Build history of the part. All positions in model axes, mm. A direction names the side the tool comes from. Give positions to 0.01 mm unless a question says otherwise; leave off trailing zeros. Order: outer loops, then holes, each group sorted by start corner. A loop starts at its lowest first (then second) coordinate and runs counter-clockwise, first axis right, second up. Notation, with made-up numbers: (61.5, 5.25) -> (79.5, 5.25) arc R11 ccw to (79.5, 25.25) -> close; hole circle Ø6 at (33, 40). An arc over 180 degrees is marked (long way). One line per question, with ' | ' between items. Start each with the question number.
(1) Which spindle directions (+Z, -Z, +X, -X, +Y, -Y) get a long thin tool onto all of the face, cutting with end or side? Do faces 4 (the face through (-378.557, 220, -53)), 5 (the face through (-403.957, 307, -329)), 6 (the face through (262, 68.014, -329)), 7 (the face through (201, -474.911, -329)), 8 (the face through (-365.857, 299, -543)). Say none if no direction does.
(2) Cut at A-A (z = -505). Give the cut face in (x, y).
(3) Cut at D-D (y = -302). Give the cut face in (x, z) (3 decimals).
(4) Cut at B-B (y = 164). Give the cut face in (x, z) (3 decimals), then the cut area to 3 significant figures.
(5) Cut at C-C (x = 76.5). Give the cut face in (y, z) (3 decimals).
(6) Drill centre lines: L1, parallel to Z at x = -89, y = 190 (3 decimals); L2, parallel to X at y = 117.5, z = -301; L3, parallel to Y at x = -385, z = -270.5. Where is each one in solid material? Low to high. Write a range as from..to.
(7) Pull direction Y, two halves, no side cores. Call faces 1 (the face through (291, -465.386, -53)), 2 (the face through (181.619, -366, -409)), 3 (the face through (-394.432, 218, -53)): +Y half, -Y half, draft (parallel to the pull), parting line (faces both ways), or undercut.
(8) Pin check, flat tips, straight feed: pin 1 Ø8 at (x, z) = (53, -203.5) entering from -Y; pin 2 Ø11.5 at (x, z) = (208, -504) entering from +Y; pin 3 Ø6 at (y, z) = (-282, -225) entering from -X. Stop position of each tip, or through.
from build123d import *

# Parameters (mm, degrees)
F1_DEPTH  = 15.875
F3_DEPTH  = 666.75
F4_W      = 139.7
F4_H      = 266.7
F4_H_2    = 244.475
F5_DEPTH  = 25.4
F6_W      = 139.7
F6_H      = 47.625
F7_DEPTH  = 12.7
F8_W      = 139.7
F8_H      = 47.625
F9_DEPTH  = 12.7
F10_W     = 139.7
F10_H     = 266.7
F10_H_2   = 244.475
F11_DEPTH = 25.4
F12_W     = 139.7
F12_H     = 47.625
F13_DEPTH = 12.7
F14_W     = 139.7
F14_H     = 47.625
F15_DEPTH = 12.7
F17_DEPTH = 504.825
F19_DEPTH = 504.825
F21_DEPTH = 3.175


with BuildPart() as f1:
    # F0 (on Top) → F1 (new body)
    with BuildSketch(Plane.XY):
        Polygon((177.06789, 329.740763), (-419.83211, 329.740763), (-419.83211, 88.440763), (159.394409, -490.785757), (400.694409, -490.785757), (400.694409, 106.114243), align=None)
    extrude(amount=F1_DEPTH)

    # F2 (on face) → F3 (join)
    with BuildSketch(Plane(origin=(0, 0, 0), x_dir=(1, 0, 0), z_dir=(0, 0, -1))):
        Polygon((397.519409, 436.810757), (397.519409, 474.910757), (359.419409, 474.910757), (359.419409, 465.385757), (219.719409, 465.385757), (219.719409, 474.910757), (181.619409, 474.910757), (181.619409, 436.810757), (219.719409, 436.810757), (219.719409, 449.510757), (359.419409, 449.510757), (359.419409, 436.810757), (381.644409, 436.810757), align=None)
        Polygon((397.519409, -83.889243), (397.519409, 436.810757), (381.644409, 436.810757), (381.644409, -68.014243), (138.96789, -68.014243), (138.96789, -310.690763), (-365.85711, -310.690763), (-365.85711, -326.565763), (154.84289, -326.565763), (154.84289, -310.690763), (154.84289, -83.889243), (381.644409, -83.889243), align=None)
        Polygon((-365.85711, -326.565763), (-365.85711, -310.690763), (-365.85711, -288.465763), (-378.55711, -288.465763), (-378.55711, -148.765763), (-365.85711, -148.765763), (-365.85711, -110.665763), (-403.95711, -110.665763), (-403.95711, -148.765763), (-394.43211, -148.765763), (-394.43211, -288.465763), (-403.95711, -288.465763), (-403.95711, -326.565763), align=None)
    extrude(amount=F3_DEPTH)

    # F4 (on face) → F5 (cut)
    with BuildSketch(Plane(origin=(-394.43211, 0, 0), x_dir=(0, -1, 0), z_dir=(-1, 0, 0))):
        with Locations((-218.615763, -241.3)):
            Rectangle(F4_W, F4_H)
        with Locations((-218.615763, -544.5125)):
            Rectangle(F4_W, F4_H_2)
    extrude(amount=-F5_DEPTH, mode=Mode.SUBTRACT)

    # F6 (on face) → F7 (join)
    with BuildSketch(Plane.YZ.offset(-378.55711)):
        with Locations((218.615763, -398.4625)):
            Rectangle(F6_W, F6_H)
    extrude(amount=F7_DEPTH)

    # F8 (on face) → F9 (cut)
    with BuildSketch(Plane(origin=(-394.43211, 0, 0), x_dir=(0, -1, 0), z_dir=(-1, 0, 0))):
        with Locations((-218.615763, -398.4625)):
            Rectangle(F8_W, F8_H)
    extrude(amount=-F9_DEPTH, mode=Mode.SUBTRACT)

    # F10 (on face) → F11 (cut)
    with BuildSketch(Plane.XZ.offset(465.385757)):
        with Locations((289.569409, -241.3)):
            Rectangle(F10_W, F10_H)
        with Locations((289.569409, -544.5125)):
            Rectangle(F10_W, F10_H_2)
    extrude(amount=-F11_DEPTH, mode=Mode.SUBTRACT)

    # F12 (on face) → F13 (join)
    with BuildSketch(Plane(origin=(0, -449.510757, 0), x_dir=(-1, 0, 0), z_dir=(0, 1, 0))):
        with Locations((-289.569409, -398.4625)):
            Rectangle(F12_W, F12_H)
    extrude(amount=F13_DEPTH)

    # F14 (on face) → F15 (cut)
    with BuildSketch(Plane.XZ.offset(465.385757)):
        with Locations((289.569409, -398.4625)):
            Rectangle(F14_W, F14_H)
    extrude(amount=-F15_DEPTH, mode=Mode.SUBTRACT)

    # F16 (on face) → F17 (join)
    with BuildSketch(Plane.YZ.offset(-365.85711)):
        Polygon((148.765763, -422.275), (288.465763, -422.275), (310.690763, -422.275), (310.690763, -406.4), (110.665763, -406.4), (110.665763, -422.275), align=None)
    extrude(amount=F17_DEPTH)

    # F18 (on face) → F19 (join)
    with BuildSketch(Plane(origin=(0, -436.810757, 0), x_dir=(-1, 0, 0), z_dir=(0, 1, 0))):
        Polygon((-381.644409, -422.275), (-359.419409, -422.275), (-219.719409, -422.275), (-181.619409, -422.275), (-181.619409, -406.4), (-381.644409, -406.4), align=None)
    extrude(amount=F19_DEPTH)

    # F20 (on face) → F21 (join)
    with BuildSketch(Plane(origin=(0, 0, -666.75), x_dir=(1, 0, 0), z_dir=(0, 0, -1))):
        Polygon((154.84289, -323.390763), (154.84289, -326.565763), (397.519409, -326.565763), (397.519409, -83.889243), (394.344409, -83.889243), (394.344409, -323.390763), align=None)
    extrude(amount=-F21_DEPTH)


solid = f1.part
Result set:
1) face 4: none | face 5: -Z, -X, +Y, -Y | face 6: -X | face 7: -Z, +X, -X, -Y | face 8: -Z, -Y
2) outline: (-403.96, 110.67) -> (-365.86, 110.67) -> (-365.86, 148.77) -> (-403.96, 148.77) -> close; (-403.96, 288.47) -> (-365.86, 288.47) -> (-365.86, 310.69) -> (138.97, 310.69) -> (138.97, 68.01) -> (381.64, 68.01) -> (381.64, -436.81) -> (359.42, -436.81) -> (359.42, -474.91) -> (397.52, -474.91) -> (397.52, 83.89) -> (154.84, 83.89) -> (154.84, 326.57) -> (-403.96, 326.57) -> close; (181.62, -474.91) -> (219.72, -474.91) -> (219.72, -436.81) -> (181.62, -436.81) -> close
3) outline: (-29.391, 0) -> (381.644, 0) -> (381.644, -406.4) -> (181.619, -406.4) -> (181.619, -422.275) -> (381.644, -422.275) -> (381.644, -666.75) -> (397.519, -666.75) -> (397.519, 0) -> (400.694, 0) -> (400.694, 15.875) -> (-29.391, 15.875) -> close
4) outline: (-419.832, 0) -> (-394.432, 0) -> (-394.432, -107.95) -> (-378.557, -107.95) -> (-378.557, 0) -> (138.968, 0) -> (138.968, -406.4) -> (-365.857, -406.4) -> (-365.857, -374.65) -> (-381.732, -374.65) -> (-381.732, -422.275) -> (138.968, -422.275) -> (138.968, -666.75) -> (154.843, -666.75) -> (154.843, 0) -> (342.809, 0) -> (342.809, 15.875) -> (-419.832, 15.875) -> close; (394.344, -666.75) -> (397.519, -666.75) -> (397.519, -663.575) -> (394.344, -663.575) -> close | area: 33,200 mm2
5) outline: (-407.891, 0) -> (310.691, 0) -> (310.691, -406.4) -> (110.666, -406.4) -> (110.666, -422.275) -> (310.691, -422.275) -> (310.691, -666.75) -> (326.566, -666.75) -> (326.566, 0) -> (329.741, 0) -> (329.741, 15.875) -> (-407.891, 15.875) -> close
6) L1: z = -422.275..-406.4, 0..15.875 | L2: x = -403.96..-365.86, 138.97..154.84 | L3: y = 110.67..148.77, 288.47..326.57
7) face 1: -Y half | face 2: draft | face 3: undercut
8) pin 1: stops at y = 310.69 | pin 2: stops at y = 83.89 | pin 3: stops at x = 381.64
